```python
from build123d import *

# Parameters (mm, degrees)
F0_R     = 69.723
F1_DEPTH = 6.35
F2_R     = 19.05
F3_DEPTH = 25.4
F4_R     = 21.6125531476
F5_DEPTH = 3.302
F6_DEPTH = 1.778
F7_R     = 3.175
F7_R_2   = 3.3636325345
F8_DEPTH = 5.08


with BuildPart() as f1:
    # F0 (on Top) → F1 (new body)
    with BuildSketch(Plane.XY):
        Circle(F0_R)
    extrude(amount=F1_DEPTH)

    # F2 (on face) → F3 (cut)
    with BuildSketch(Plane.XY.offset(6.35)):
        Circle(F2_R)
    extrude(amount=-F3_DEPTH, mode=Mode.SUBTRACT)

    # F4 (on face) → F5 (cut)
    with BuildSketch(Plane.XY.offset(6.35)):
        Circle(F4_R)
    extrude(amount=-F5_DEPTH, mode=Mode.SUBTRACT)

    # F6 (cut): a face of the model
    f6_faces = [f1.faces().sort_by_distance(p)[0] for p in [
        (-21.001257832, 0, 3.048),
    ]]
    extrude(f6_faces, amount=-F6_DEPTH, mode=Mode.SUBTRACT)

    # F7 (on face) → F8 (join)
    with BuildSketch(Plane.XY.offset(6.35)):
        with Locations((0, 38.1)):
            Circle(F7_R)
        with Locations((0, -38.1)):
            Circle(F7_R_2)
    extrude(amount=F8_DEPTH)


solid = f1.part
```
Input: part model. Units: mm. Frame: model coordinates. A direction names the side the tool comes from. Round coordinates to 2 decimals unless told otherwise and drop trailing zeros. Loops run counter-clockwise (first coordinate to the right, second up) from the corner with the lowest first, then second, coordinate; pieces in that order, holes last. Notation, with made-up numbers: (20.25, -9) - (33.25, -9) arc R5 cw to (33.25, -3) - close; hole circle Ø11 at (7, 38.5). An arc over 180 degrees is marked (long way). One line per item, written item: value. Start each with the question number.
(1) Ray query, line 1 (Y direction, x = 0, z = 2.85); line 2 (Z direction, x = -26, y = 14.5); line 3 (Y direction, x = -17.5, z = 3.5). Return the intervals inside material, ascending. Write a range as [from, to].
(2) Section C-C, the plane z = 3.75. Return loops of the section in (x, y), plus the area to 3 significant figures.
(3) Section B-B, the plane y = 0. Return loops of the section in (x, z), plus the area to 3 significant figures.
(4) Access query for faces 4 (the cylindrical face through (-9.08, 69.13, 3.13)), 5 (the cylindrical face through (-0.69, 35, 8.85)). Directions: +Z, -Z, +X, -X, +Y, -Y. A direction counts if a zero-diameter tool reaches every point of the face in a straight line with its end or side. Return the directions, or none.
(5) Section A-A, the plane x = 0. Return loops of the section in (y, z) (3 decimals), plus the area to 3 significant figures.
(6) Draft query along X for faces 1 (the cylindrical face through (-0.438, -34.765, 8.854)), 2 (the flat face through (0, 38, 11.43)), 3 (the cylindrical face through (-15.12, -11.59, 0.64)). Return one class per face: +X half, -X half, draft (parallel to the pull), parting line (faces both ways), or undercut.
(7) Section D-D, the plane y = -38.1. Return loops of the section in (x, z).
(8) Contact query for flat-ended pins moving along their axis: P1, Ø6, axis at y = 8.5, z = 5, coming from the +X side; P2, Ø5, axis at x = -9, z = 2.5, coming from the +Y side; P3, Ø1, axis at y = -24, z = 5, coming from the +X side. Output: stop coordinate, or through.
Results below:
1. line 1: [-69.72, -21.61], [21.61, 69.72]
1. line 2: [0, 6.35]
1. line 3: [-67.49, -12.68], [12.68, 67.49]
2. outline: circle Ø139.45 at (0, 0); hole circle Ø43.23 at (0, 0)
2. area: 13,800 mm^2
3. outline: (-69.72, 0) - (-19.05, 0) - (-19.05, 1.27) - (-21.61, 1.27) - (-21.61, 6.35) - (-69.72, 6.35) - close; (19.05, 0) - (69.72, 0) - (69.72, 6.35) - (21.61, 6.35) - (21.61, 1.27) - (19.05, 1.27) - close
3. area: 618 mm^2
4. face 4: +Z, -Z
4. face 5: +Z
5. outline: (-69.723, 0) - (-19.05, 0) - (-19.05, 1.27) - (-21.613, 1.27) - (-21.613, 6.35) - (-34.736, 6.35) - (-34.736, 11.43) - (-41.464, 11.43) - (-41.464, 6.35) - (-69.723, 6.35) - close; (19.05, 0) - (69.723, 0) - (69.723, 6.35) - (41.275, 6.35) - (41.275, 11.43) - (34.925, 11.43) - (34.925, 6.35) - (21.613, 6.35) - (21.613, 1.27) - (19.05, 1.27) - close
5. area: 684 mm^2
6. face 1: parting line
6. face 2: draft
6. face 3: undercut
7. outline: (-58.39, 0) - (58.39, 0) - (58.39, 6.35) - (3.36, 6.35) - (3.36, 11.43) - (-3.36, 11.43) - (-3.36, 6.35) - (-58.39, 6.35) - close
8. P1: x = 69.51
8. P2: y = 69.42
8. P3: x = 65.64
